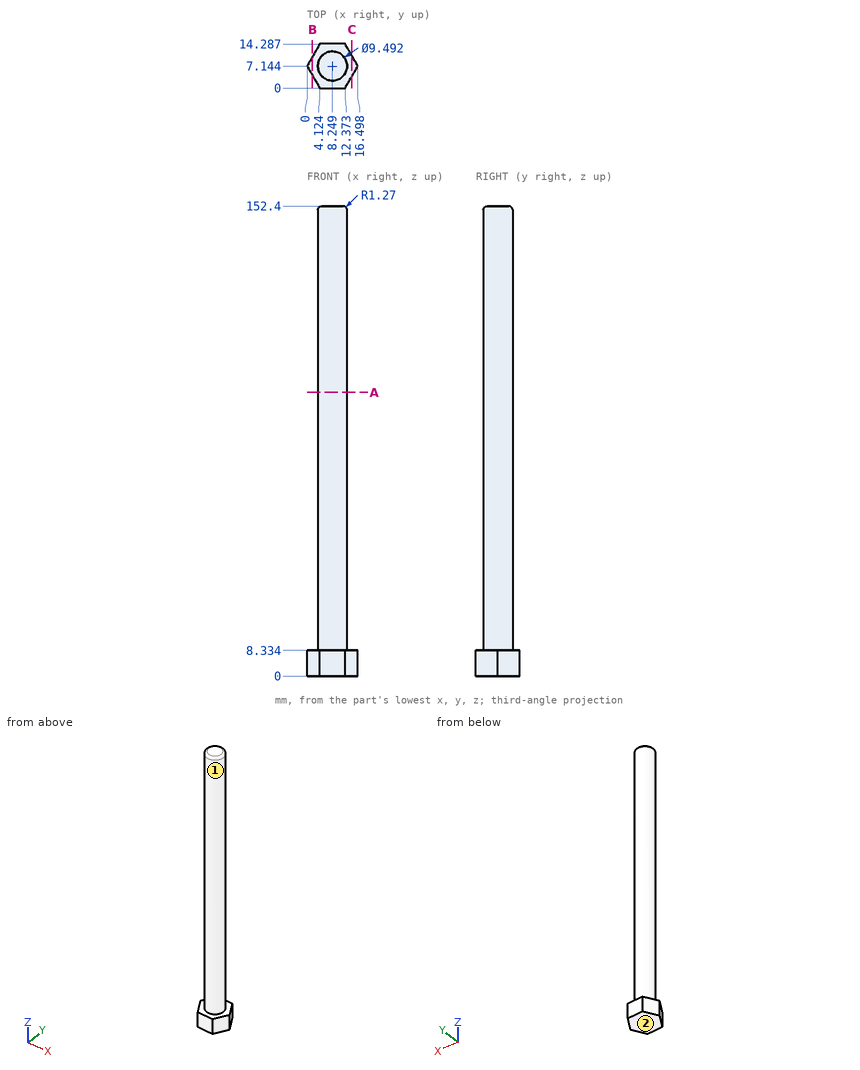
Job drawing, mm, ordinate dimensions from the low corner. One solid piece. A direction names the side the tool comes from. Round coordinates to 2 decimals unless told otherwise and drop trailing zeros. Loops run counter-clockwise (first coordinate to the right, second up) from the corner with the lowest first, then second, coordinate; pieces in that order, holes last. Notation, with made-up numbers: (45.25, 20.25) -> (82.25, 20.25) arc R22 ccw to (82.25, 43.25) -> close; hole circle Ø7 at (-17, 3). An arc over 180 degrees is marked (long way). One line per item, written item: value. Start each with the question number.
Q1. Cut at B-B on x = 1.75. List the corners of the cut face in (y, z) (1 decimal).
Q2. Cut at A-A on z = 92. List the corners of the cut face in (x, y) (1 decimal).
Q3. Cut at C-C on x = 14.5. List the corners of the cut face in (y, z) (1 decimal).
Q4. 3-axis set-ups, long thin cutter, end or side, ignore diameter. For the marked faces 1 and 2: which of +Z, -Z, +X, -X, +Y, -Y reach the whole face in a straight line?
Q5. Drop flat-ended pins along their axis: pin 1 Ø2 at (y, z) = (7.5, 98.5) entering from -X; pin 2 Ø8 at (x, z) = (9, 33) entering from +Y; pin 3 Ø5 at (y, z) = (11.5, 113) entering from +X. Give the stop position or say it passes through.
Q6. Probe line 1 along Z through (x, y) = (4.5, 11) (1 decimal); line 2 along Y through (x, z) = (8.75, 19) (1 decimal); line 3 along X through (y, z) = (5.75, 64) (1 decimal). List the from-to ranges inside material, lowest first.
Computed:
1. outline: (4.1, 0) -> (10.2, 0) -> (10.2, 8.3) -> (4.1, 8.3) -> close
2. outline: circle Ø9.5 at (8.2, 7.1)
3. outline: (3.7, 0) -> (10.6, 0) -> (10.6, 8.3) -> (3.7, 8.3) -> close
4. face 1: +Z
4. face 2: -Z, +X, -X, +Y, -Y
5. pin 1: x = 3.5
5. pin 2: y = 11.89
5. pin 3: x = 12.62
6. line 1: 0 to 8.3
6. line 2: 2.4 to 11.9
6. line 3: 3.7 to 12.8
